For this review, take the finished solid that the model builds, in its own axes (mm). Coordinates: 2 decimals unless noted, no trailing zeros. Order: outer loops, then holes, each group sorted by start corner. A loop starts at its lowest first (then second) coordinate and runs counter-clockwise, first axis right, second up. Notation, with made-up numbers: (59, -12) -> (74, -12) arc R18 ccw to (74, -7) -> close; hole circle Ø11 at (-23, 81.25). An arc over 180 degrees is marked (long way). Answer as a JSON object with one key per item and string values. Group by question number.
1) Add section A-A, the plane y = 0.65. Write out the cut boundary in (x, z), then the cut area to 3 significant figures.
2) Wall thickness on L1, parallel to Y at x = 0, z = 18.5; L2, parallel to X at y = 0.25, z = 16.5; L3, parallel to X at y = 0.65, z = 11.5: over which ranges is each line inside the solid? List them lowest first.
3) For pin 1 (1.8 mm diameter, centred on x = 0, y = 0, fed in from +Z); pin 2 (1 mm diameter, centred on x = 1, z = 12, fed in from -Y), all flat-tipped, find the tip position at first contact; note any pin that passes through.
4) Add section C-C, the plane z = 24. Write out the cut boundary in (x, y), then the cut area to 3 significant figures.
5) Add section B-B, the plane x = 0. Write out the cut boundary in (y, z), then the cut area to 3 significant figures.
from build123d import *

# Parameters (mm, degrees)
DOWEL_BODY_DEPTH = 38


with BuildPart() as part:
    # Sketch1 → dowel_body (new body)
    with BuildSketch(Plane.XY):
        with BuildLine():
            Line((-0.4, -1.600781059), (-0.4, -0.916515139))
            ThreePointArc((-0.4, -0.916515139), (-0.547722558, 0.836660027), (1, 0))
            ThreePointArc((1, 0), (0.836660027, -0.547722558), (0.4, -0.916515139))
            Line((0.4, -0.916515139), (0.4, -1.600781059))
            ThreePointArc((0.4, -1.600781059), (1.30048068, -1.015504801), (1.65, 0))
            ThreePointArc((1.65, 0), (-1.015504801, 1.30048068), (-0.4, -1.600781059))
        make_face()
    extrude(amount=DOWEL_BODY_DEPTH)


solid = part.part
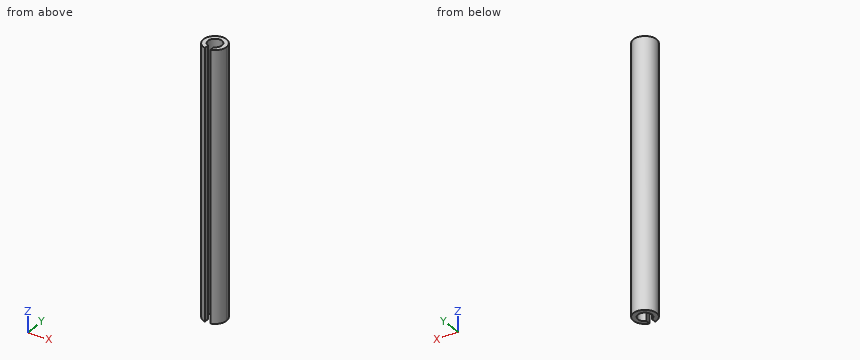
Output values:
{
 "1": {"outline": "(-1.52, 0) -> (-0.76, 0) -> (-0.76, 38) -> (-1.52, 38) -> close; (0.76, 0) -> (1.52, 0) -> (1.52, 38) -> (0.76, 38) -> close", "area": "57.5 mm²"},
 "2": {"L1": "y = 1 to 1.65", "L2": "x = -1.63 to -0.97, 0.97 to 1.63", "L3": "x = -1.52 to -0.76, 0.76 to 1.52"},
 "3": {"pin 1": "passes through", "pin 2": "stops at y = -1.57"},
 "4": {"outline": "(-0.4, -1.6) -> (-0.4, -0.92) arc R1 cw (long way) to (0.4, -0.92) -> (0.4, -1.6) arc R1.65 ccw (long way) to start", "area": "4.88 mm²"},
 "5": {"outline": "(1, 0) -> (1.65, 0) -> (1.65, 38) -> (1, 38) -> close", "area": "24.7 mm²"}
}
